The figure shows three views and two pictorial views of one solid part (mm, origin at its lowest corner). Answer the questions. Round coordinates to 2 decimals unless told otherwise and drop trailing zeros. Order: outer loops, then holes, each group sorted by start corner. A loop starts at its lowest first (then second) coordinate and runs counter-clockwise, first axis right, second up. Notation, with made-up numbers: (-16.5, -3.5) -> (22.5, -3.5) arc R31 cw to (22.5, 25.5) -> close; hole circle Ø3 at (-10, 83). An arc over 180 degrees is marked (long way). Answer as a JSON object with one key per item and string values. Group by question number.
Item 1: Section A-A, the plane z = 0.45 is taken. Write down the section's boundary in (x, y), plus the area to 3 significant figures.
Item 2: Section B-B, the plane x = 12.5 is taken. Write down the section's boundary in (y, z), plus the area to 3 significant figures.
Item 3: Consider probe 1 along X at (y, z) = (10, 1). Determine where the line is inside the solid, lowest interval first. Write a range as from..to.
Item 4: Given P1, Ø0.6, axis at x = 19, z = 1, coming from the -Y side; P2, Ø0.6, axis at y = 14.5, z = 1, coming from the -X side; P3, Ø2, axis at x = 31.5, y = 38.5, coming from the -Z side, each flat-ended and moving along its own axis, determine where each tip first touches the part or whether it passes through.
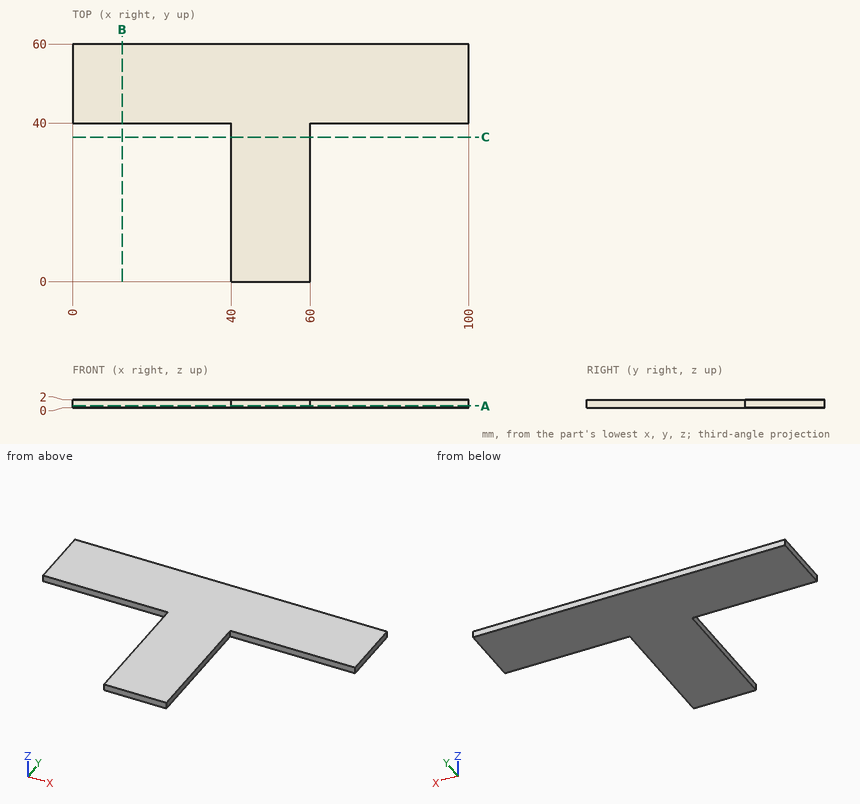
Values found:
{
 "1": {"outline": "(0, 40) -> (40, 40) -> (40, 0) -> (60, 0) -> (60, 40) -> (100, 40) -> (100, 60) -> (0, 60) -> close", "area": "2,800 mm2"},
 "2": {"outline": "(40, 0) -> (60, 0) -> (60, 2) -> (40, 2) -> close", "area": "40.0 mm2"},
 "3": {"probe 1": "40..60"},
 "4": {"P1": "y = 40", "P2": "x = 40", "P3": "through"}
}
